```python
from build123d import *

# Parameters (mm, degrees)
SKETCH1_W           = 60
SKETCH1_H           = 60
SKETCH1_R           = 3.175
BOSS_EXTRUDE1_DEPTH = 2
SKETCH3_R           = 2
CUT_EXTRUDE2_DEPTH  = 85.947042326


with BuildPart() as part:
    # Sketch1 → Boss-Extrude1 (new, symmetric)
    with BuildSketch(Plane.XY):
        with Locations((30, 30)):
            Rectangle(SKETCH1_W, SKETCH1_H)
        with Locations((15, 30)):
            Circle(SKETCH1_R, mode=Mode.SUBTRACT)
        with Locations((45, 30)):
            Circle(SKETCH1_R, mode=Mode.SUBTRACT)
    extrude(amount=BOSS_EXTRUDE1_DEPTH, both=True)

    # Cut-Extrude1 cone 1 section (through the dimple's axis) → Cut-Extrude1 (revolve, cut)
    with BuildSketch(Plane(origin=(15, 30, 2), x_dir=(0, -1, 0), z_dir=(1, 0, 0))):
        Polygon((0, 0), (6.9088, 0), (0, 6.9088), align=None)
    revolve(axis=Axis((15, 30, 2), (0, 0, -1)), mode=Mode.SUBTRACT)

    # Cut-Extrude1 cone 2 section (through the dimple's axis) → Cut-Extrude1 cone 2 (revolve, cut)
    with BuildSketch(Plane(origin=(45, 30, 2), x_dir=(0, -1, 0), z_dir=(1, 0, 0))):
        Polygon((0, 0), (6.9088, 0), (0, 6.9088), align=None)
    revolve(axis=Axis((45, 30, 2), (0, 0, -1)), mode=Mode.SUBTRACT)

    # Sketch3 → Cut-Extrude2 (cut, through all)
    with BuildSketch(Plane.XY.offset(2)):
        with Locations((22, 14)):
            Circle(SKETCH3_R)
        with Locations((38, 14)):
            Circle(SKETCH3_R)
        with Locations((38, 46)):
            Circle(SKETCH3_R)
        with Locations((22, 46)):
            Circle(SKETCH3_R)
    extrude(amount=-CUT_EXTRUDE2_DEPTH, mode=Mode.SUBTRACT)


solid = part.part
```
The model under review builds one solid part; all positions refer to its coordinate system, in mm. Coordinates: 2 decimals unless noted, no trailing zeros. Write each loop counter-clockwise with the first axis right and the second up, starting at its lowest first coordinate (ties: lowest second). Pieces come first, ordered by that corner, then holes. Notation, with made-up numbers: (87, -28) - (120, -28) arc R18 cw to (120, -24) - close; hole circle Ø7 at (49, 0). An arc over 180 degrees is marked (long way). Write item = value, one per line.
(1) For line 1 (Y direction, x = 38, z = -0.35); line 2 (X direction, y = 30, z = -1.9) (3 decimals); line 3 (Y direction, x = 15, z = -1.75) (3 decimals), list the stretches that pass through material, from the lowest coordinate up. Write a range as [from, to].
Result sheet:
line_1 = [0, 12], [16, 44], [48, 60]
line_2 = [0, 11.825], [18.175, 41.825], [48.175, 60]
line_3 = [0, 26.825], [33.175, 60]
(2) Mouldability with a two-part tool opening along Y and no side actions: class faces 1 (the face through (41.67, 30.44, -1.55)), 2 (the face through (30, 30, 2)), 3 (the face through (30, 0, 0)), 4 (the face through (12.732, 32.474, -1.553)) as pulls with the +Y half, pulls with the -Y half, needs draft (parallel to the pull), parting line crosses it, or undercut.
Result sheet:
face_1 = undercut
face_2 = needs draft
face_3 = pulls with the -Y half
face_4 = undercut
(3) Consider section B-B, the plane y = 30. Give the boundary of the cut face in (x, z) (3 decimals).
Result sheet:
outline = (0, -2) - (11.825, -2) - (11.825, -1.734) - (8.091, 2) - (0, 2) - close; (18.175, -2) - (41.825, -2) - (41.825, -1.734) - (38.091, 2) - (21.909, 2) - (18.175, -1.734) - close; (48.175, -2) - (60, -2) - (60, 2) - (51.909, 2) - (48.175, -1.734) - close
(4) For P1, Ø6.5, axis at x = 38, y = 14, coming from the -Z side; P2, Ø4, axis at x = 45, y = 30, coming from the -Z side, all flat-tipped, find the tip position at first contact; note any pin that passes through.
Result sheet:
P1 = -2
P2 = through
(5) Consider section A-A, the plane x = 45. Give the boundary of the cut face in (y, z) (3 decimals), then the cut area to 3 significant figures.
Result sheet:
outline = (0, -2) - (26.825, -2) - (26.825, -1.734) - (23.091, 2) - (0, 2) - close; (33.175, -2) - (60, -2) - (60, 2) - (36.909, 2) - (33.175, -1.734) - close
area = 201 mm^2
(6) Consider section C-C, the plane z = -0.35. Give the boundary of the cut face in (x, y), then the cut area to 3 significant figures.
Result sheet:
outline = (0, 0) - (60, 0) - (60, 60) - (0, 60) - close; hole circle Ø9.12 at (15, 30); hole circle Ø4 at (22, 14); hole circle Ø4 at (22, 46); hole circle Ø4 at (38, 14); hole circle Ø4 at (38, 46); hole circle Ø9.12 at (45, 30)
area = 3,420 mm^2
(7) Consider section D-D, the plane y = 46. Give the boundary of the cut face in (x, z).
Result sheet:
outline = (0, -2) - (20, -2) - (20, 2) - (0, 2) - close; (24, -2) - (36, -2) - (36, 2) - (24, 2) - close; (40, -2) - (60, -2) - (60, 2) - (40, 2) - close
